from build123d import *
from build123d.topology import SkipClean

# Parameters (mm, degrees)
BOSS_EXTRUDE1_DEPTH = 19
SKETCH2_W           = 44.8
SKETCH2_H           = 35
BOSS_EXTRUDE2_DEPTH = 2
CUT_EXTRUDE1_START  = -2
SKETCH3_R           = 20.8
CUT_EXTRUDE1_DEPTH  = 2
SKETCH4_R           = 1
CUT_EXTRUDE2_DEPTH  = 2
FILLET1_R           = 8
SKETCH5_W           = 18.8
SKETCH5_H           = 6.055148909
SKETCH5_H_2         = 6.944851091
CUT_EXTRUDE3_DEPTH  = 47
FILLET2_START       = -23
FILLET2_DEPTH       = 46


with BuildPart() as part:
    # Sketch1 → Boss-Extrude1 (new body)
    with BuildSketch(Plane(origin=(0, 0, 0), x_dir=(1, 0, 0), z_dir=(0, 1, 0))):
        with BuildLine():
            Line((-22.4, 0), (-20.8, 0))
            ThreePointArc((-20.8, 0), (0, 20.8), (20.8, 0))
            Line((20.8, 0), (22.4, 0))
            ThreePointArc((22.4, 0), (0, 22.4), (-22.4, 0))
        make_face()
    extrude(amount=BOSS_EXTRUDE1_DEPTH)

    # Sketch2 → Boss-Extrude2 (add)
    with BuildSketch(Plane.XZ):
        with Locations((0, -17.5)):
            Rectangle(SKETCH2_W, SKETCH2_H)
    extrude(amount=BOSS_EXTRUDE2_DEPTH)

    # Sketch3 → Cut-Extrude1 (cut)
    with SkipClean():  # the faces are left unmerged after this step: merging them gives an invalid solid
        with BuildSketch(Plane(origin=(0, 0, 0), x_dir=(1, 0, 0), z_dir=(0, 1, 0)).offset(CUT_EXTRUDE1_START)):
            Circle(SKETCH3_R)
        extrude(amount=CUT_EXTRUDE1_DEPTH, mode=Mode.SUBTRACT)
    add(part.part.scale(1), mode=Mode.REPLACE)  # the faces are merged on a copy

    # Sketch4 → Cut-Extrude2 (cut)
    with BuildSketch(Plane(origin=(0, 0, 0), x_dir=(1, 0, 0), z_dir=(0, 1, 0))):
        with Locations(Location((-8, 32, 0), (0, 0, 270))):
            Circle(SKETCH4_R)
        with Locations(Location((8, 32, 0), (0, 0, 90))):
            Circle(SKETCH4_R)
    extrude(amount=-CUT_EXTRUDE2_DEPTH, mode=Mode.SUBTRACT)

    # Fillet1
    fillet1_edges = [part.edges().sort_by_distance(p)[0] for p in [
        (-22.4, -1, -35),
        (22.4, -1, -35),
    ]]
    fillet(fillet1_edges, radius=FILLET1_R)

    # Sketch5 → Cut-Extrude3 (cut)
    with BuildSketch(Plane.ZY.offset(22.4)):
        with Locations((-11.4, 13.972425546)):
            Rectangle(SKETCH5_W, SKETCH5_H)
        with Locations((-11.4, 5.472425546)):
            Rectangle(SKETCH5_W, SKETCH5_H_2)
    extrude(amount=-CUT_EXTRUDE3_DEPTH, mode=Mode.SUBTRACT)

    # Fillet2: read off the stored shape, not the designer's step
    # Fillet2 outline → Fillet2 (cut)
    with BuildSketch(Plane.YZ.offset(FILLET2_START)):
        with BuildLine():
            Line((1, 0), (-2, 0))
            Line((-2, 0), (-2, -3))
            ThreePointArc((-2, -3), (-1.121320344, -0.878679656), (1, 0))
        make_face()
    extrude(amount=FILLET2_DEPTH, mode=Mode.SUBTRACT)


solid = part.part
The listing builds one solid part. Answer for the finished solid, in the listing's coordinates (mm). A direction names the side the tool comes from. Coordinates: 2 decimals unless noted, no trailing zeros. Write each loop counter-clockwise with the first axis right and the second up, starting at its lowest first coordinate (ties: lowest second). Pieces come first, ordered by that corner, then holes. Notation, with made-up numbers: M 2,42 L 21,42 A18 cw 21,75 Z; hole C 57,88 d2. An arc over 180 degrees is marked long. Use one line per item in the form item = value.
Item 1: The mould has two halves that part along Y. Classify faces 4 (the face through (0, -2, -22)), 5 (the face through (0, 0, -25)), 6 (the face through (-22, 5, -2)): released by +Y, released by -Y, zero draft, split by the parting line, or undercut.
Model answer:
face_4 = released by -Y
face_5 = released by +Y
face_6 = undercut
Item 2: Find section C-C, the plane x = -17. Give the vertices of the cut face in (y, z) (3 decimals).
Model answer:
outline = M -2,-34.566 L 0,-34.566 L 0,-14.586 L 2,-14.586 L 2,-11.985 L -2,-11.985 Z; M 8.945,-14.586 L 10.945,-14.586 L 10.945,-11.985 L 8.945,-11.985 Z; M 17,-14.586 L 19,-14.586 L 19,-11.985 L 17,-11.985 Z
Item 3: Find the intervals of material crossed by probe 1 along Y at (x, z) = (17, -13); probe 2 along X at (y, z) = (-1, -32) (3 decimals); probe 3 along Y at (x, z) = (5, -32), in increasing order.
Model answer:
probe_1 = -2 to 2, 8.94 to 10.94, 17 to 19
probe_2 = -20.645 to -9, -7 to 7, 9 to 20.645
probe_3 = -2 to 0
Item 4: Find section D-D, the plane z = -32. Give the vertices of the cut face in (x, y) (3 decimals).
Model answer:
outline = M -20.645,-2 L -9,-2 L -9,0 L -20.645,0 Z; M -7,-2 L 7,-2 L 7,0 L -7,0 Z; M 9,-2 L 20.645,-2 L 20.645,0 L 9,0 Z
Item 5: Find section A-A, the plane y = 4.25. Give the vertices of the cut face in (x, z).
Model answer:
outline = M -22.4,0 A22.4 ccw -22.31,-2 L -20.7,-2 A20.8 cw -20.8,0 Z; M -8.31,-20.8 A22.4 ccw 8.31,-20.8 Z; M 20.7,-2 L 22.31,-2 A22.4 ccw 22.4,0 L 20.8,0 A20.8 cw Z
Item 6: Given P1, Ø10, axis at y = 9.5, z = -14.5, coming from the -X side; P2, Ø1, axis at y = 2, z = -18.5, coming from the -X side; P3, Ø1.3, axis at x = 21.5, y = 5.5, coming from the -Z side, each flat-ended and moving along its own axis, determine where each tip first touches the part or whether it passes through.
Model answer:
P1 = -20.29
P2 = -13.33
P3 = -2
Item 7: Find section B-B, the plane z = -5. Give the vertices of the cut face in (x, y), plus the area to 3 significant figures.
Model answer:
outline = M -22.4,-2 L -20.19,-2 L -20.19,2 L -21.83,2 L -21.83,0 L -22.4,0 Z; M -21.83,8.94 L -20.19,8.94 L -20.19,10.94 L -21.83,10.94 Z; M -21.83,17 L -20.19,17 L -20.19,19 L -21.83,19 Z; M 20.19,-2 L 22.4,-2 L 22.4,0 L 21.83,0 L 21.83,2 L 20.19,2 Z; M 20.19,8.94 L 21.83,8.94 L 21.83,10.94 L 20.19,10.94 Z; M 20.19,17 L 21.83,17 L 21.83,19 L 20.19,19 Z
area = 28.6 mm2
Item 8: For faces 1 (the face through (0, 5, -20.8)), 2 (the face through (-21.5, -1.14, -0.9)), 3 (the face through (21, 14, -2)), determine the directions among +Z, -Z, +X, -X, +Y, -Y from which every point of the face is accessible in a straight line to the end or side of a thin tool.
Model answer:
face_1 = +Z, +X, -X
face_2 = +Z, +X, -X, -Y
face_3 = -Z, +X, -X
